Part model, mm, in its own coordinate system. Round coordinates to 2 decimals unless told otherwise and drop trailing zeros. Loops run counter-clockwise (first coordinate to the right, second up) from the corner with the lowest first, then second, coordinate; pieces in that order, holes last.
(1) Flat gauge pins, fed straight in: pin 1 (3 mm diameter, centred on x = -21, z = 5.5, fed in from +Y); pin 2 (5.5 mm diameter, centred on x = -149.225, y = 0, fed in from -Z); pin 3 (2 mm diameter, centred on x = 31, z = 0.5, fed in from +Y); pin 4 (4 mm diameter, centred on x = -106, z = -8.5, fed in from +Y). Where does each tip first touch, or does it go through?
(2) Cut at B-B on z = 0. List the corners of the cut face in (x, y) (3 decimals).
(3) Probe probe 1 along X at (y, z) = (0, -19.9) (3 decimals); probe 2 along Z at (x, y) = (75.5, 0.5); probe 3 along Y at (x, z) = (16.5, -14). List the from-to ranges inside material, lowest first.
(4) Cut at C-C on y = 13.5. List the corners of the cut face in (x, z) (3 decimals).
(5) Cut at A-A on y = 0. List the corners of the cut face in (x, z) (3 decimals), then the cut area to 3 significant figures.
(6) Cut at D-D on x = 26. List the corners of the cut face in (y, z).
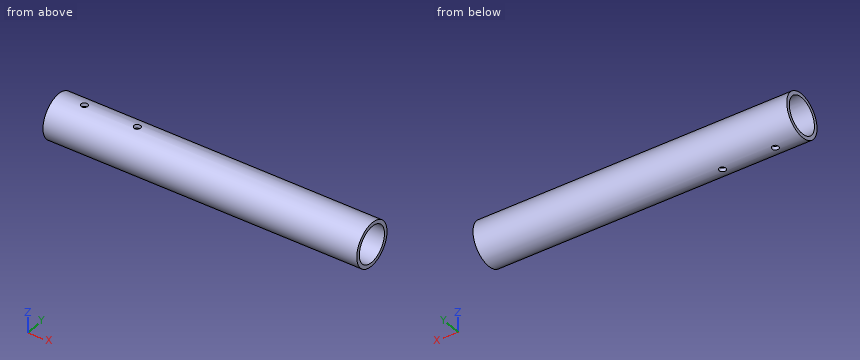
from build123d import *

# Parameters (mm, degrees)
SKETCH1_R                = 21.082
SKETCH1_R_2              = 17.526
BOSS_EXTRUDE1_DEPTH      = 127
BOSS_EXTRUDE1_DEPTH_BACK = 174.625
SKETCH2_R                = 3.175
CUT_EXTRUDE1_DEPTH       = 22.082
CUT_EXTRUDE1_DEPTH_BACK  = 22.082


with BuildPart() as part:
    # Sketch1 → Boss-Extrude1 (new body, two sides)
    with BuildSketch(Plane(origin=(0, 0, 0), x_dir=(0, 0, -1), z_dir=(1, 0, 0))) as boss_extrude1_sk:
        Circle(SKETCH1_R)
        Circle(SKETCH1_R_2, mode=Mode.SUBTRACT)
    extrude(amount=BOSS_EXTRUDE1_DEPTH)
    extrude(boss_extrude1_sk.sketch, amount=-BOSS_EXTRUDE1_DEPTH_BACK)

    # Sketch2 → Cut-Extrude1 (cut, two sides)
    with BuildSketch(Plane.XY) as cut_extrude1_sk:
        with Locations((-98.425, 0)):
            Circle(SKETCH2_R)
        with Locations((-149.225, 0)):
            Circle(SKETCH2_R)
    extrude(amount=CUT_EXTRUDE1_DEPTH, mode=Mode.SUBTRACT)
    extrude(cut_extrude1_sk.sketch, amount=-CUT_EXTRUDE1_DEPTH_BACK, mode=Mode.SUBTRACT)


solid = part.part
Final values:
1. pin 1: stops at y = 20.7
1. pin 2: passes through
1. pin 3: stops at y = 21.08
1. pin 4: stops at y = 20.05
2. outline: (-174.625, -21.082) - (127, -21.082) - (127, -17.526) - (-174.625, -17.526) - close; (-174.625, 17.526) - (127, 17.526) - (127, 21.082) - (-174.625, 21.082) - close
3. probe 1: x = -174.625 to -152.4, -146.05 to -101.6, -95.25 to 127
3. probe 2: z = -21.08 to -17.52, 17.52 to 21.08
3. probe 3: y = -15.76 to -10.54, 10.54 to 15.76
4. outline: (-174.625, -16.193) - (127, -16.193) - (127, -11.176) - (-174.625, -11.176) - close; (-174.625, 11.176) - (127, 11.176) - (127, 16.193) - (-174.625, 16.193) - close
5. outline: (-174.625, -21.082) - (-152.4, -21.082) - (-152.4, -17.526) - (-174.625, -17.526) - close; (-174.625, 17.526) - (-152.4, 17.526) - (-152.4, 21.082) - (-174.625, 21.082) - close; (-146.05, -21.082) - (-101.6, -21.082) - (-101.6, -17.526) - (-146.05, -17.526) - close; (-146.05, 17.526) - (-101.6, 17.526) - (-101.6, 21.082) - (-146.05, 21.082) - close; (-95.25, -21.082) - (127, -21.082) - (127, -17.526) - (-95.25, -17.526) - close; (-95.25, 17.526) - (127, 17.526) - (127, 21.082) - (-95.25, 21.082) - close
5. area: 2,050 mm2
6. outline: circle Ø42.16 at (0, 0); hole circle Ø35.05 at (0, 0)
